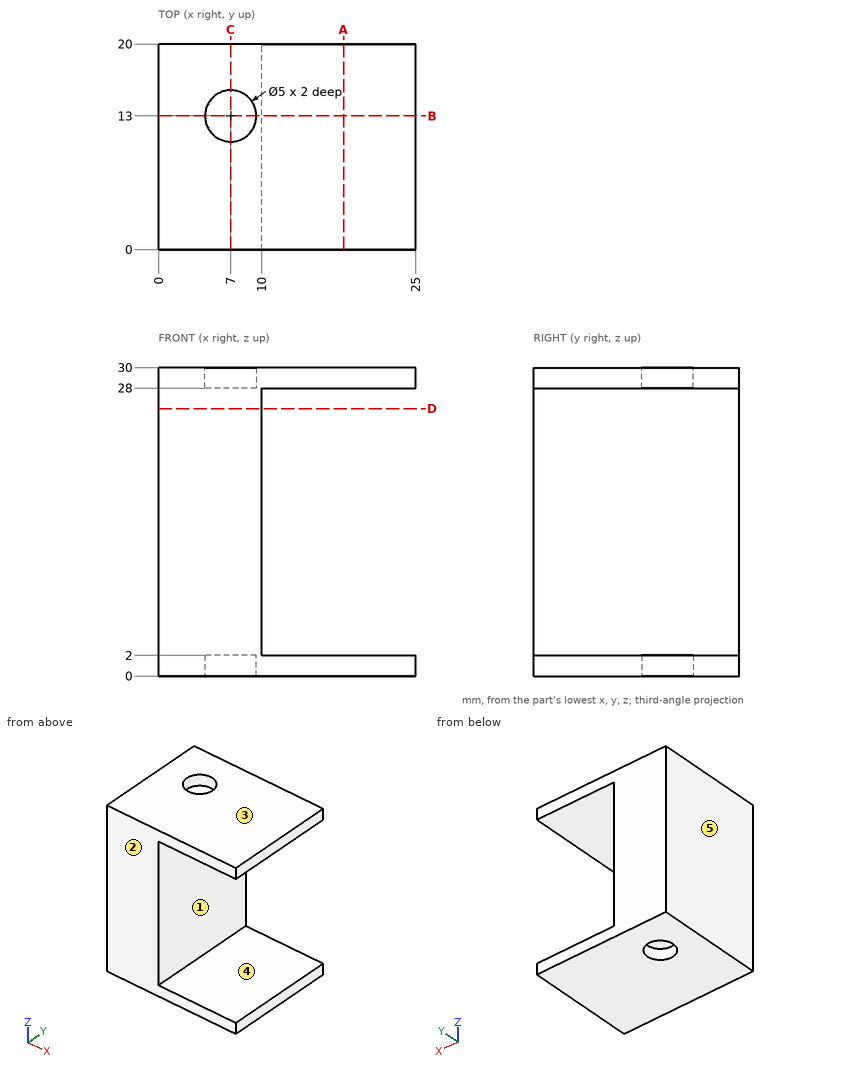
Source: three-view drawing plus pictorial views. Frame: mm from the lowest corner of the part. A direction names the side the tool comes from. Coordinates: 2 decimals unless noted, no trailing zeros. Loops run counter-clockwise (first coordinate to the right, second up) from the corner with the lowest first, then second, coordinate; pieces in that order, holes last. Notation, with made-up numbers: (-5.75, -26) -> (53.25, -26) arc R30 ccw to (53.25, 1) -> close; hole circle Ø11 at (-5, 52.25). An arc over 180 degrees is marked (long way). Answer in a Markdown table with one row per item. Add a question column.
Q1. Ray query, line 1 along Z through (x, y) = (24, 12.75); line 2 along Y through (x, z) = (7, 29.4); line 3 along X through (y, z) = (18.25, 22). Return the intervals inside material, ascending.
Q2. Section C-C on x = 7. Return the cut outline in (y, z).
Q3. Reachability of the marked faces 4 and 5 from +Z, -Z, +X, -X, +Y, -Y: full face, straight path, thin tool, end or side. Return the list, or none.
Q4. Pull-direction query (Z, two-part tool) for the marked faces 1, 2 and 3; classes: pulls with the +Z half, pulls with the -Z half, needs draft (parallel to the pull), parting line crosses it, or undercut.
Q5. Section A-A on x = 18. Return the cut outline in (y, z), and give its area (3 significant figures).
Q6. Section B-B on y = 13. Return the cut outline in (x, z), and give its area (3 significant figures).
Q7. Section D-D on z = 26. Return the cut outline in (x, y), and give its area (3 significant figures).
Q8. Contact query for flat-ended pins moving along their axis: pin 1 Ø6.5 at (x, y) = (7, 13) entering from -Z; pin 2 Ø10 at (y, z) = (8.5, 10.5) entering from +X. Output: stop coordinate, or through.
Computed values:
| question | item | result |
|---|---|---|
| 1 | line 1 | z = 0 to 2, 28 to 30 |
| 1 | line 2 | y = 0 to 10.5, 15.5 to 20 |
| 1 | line 3 | x = 0 to 10 |
| 2 | outline | (0, 0) -> (10.5, 0) -> (10.5, 2) -> (15.5, 2) -> (15.5, 0) -> (20, 0) -> (20, 30) -> (15.5, 30) -> (15.5, 28) -> (10.5, 28) -> (10.5, 30) -> (0, 30) -> close |
| 3 | face 4 | +X, +Y, -Y |
| 3 | face 5 | +Z, -Z, -X, +Y, -Y |
| 4 | face 1 | undercut |
| 4 | face 2 | needs draft |
| 4 | face 3 | pulls with the +Z half |
| 5 | outline | (0, 0) -> (20, 0) -> (20, 2) -> (0, 2) -> close; (0, 28) -> (20, 28) -> (20, 30) -> (0, 30) -> close |
| 5 | area | 80.0 mm^2 |
| 6 | outline | (0, 0) -> (4.5, 0) -> (4.5, 2) -> (9.5, 2) -> (9.5, 0) -> (25, 0) -> (25, 2) -> (10, 2) -> (10, 28) -> (25, 28) -> (25, 30) -> (9.5, 30) -> (9.5, 28) -> (4.5, 28) -> (4.5, 30) -> (0, 30) -> close |
| 6 | area | 340 mm^2 |
| 7 | outline | (0, 0) -> (10, 0) -> (10, 20) -> (0, 20) -> close |
| 7 | area | 200 mm^2 |
| 8 | pin 1 | stops at z = 0 |
| 8 | pin 2 | stops at x = 10 |
